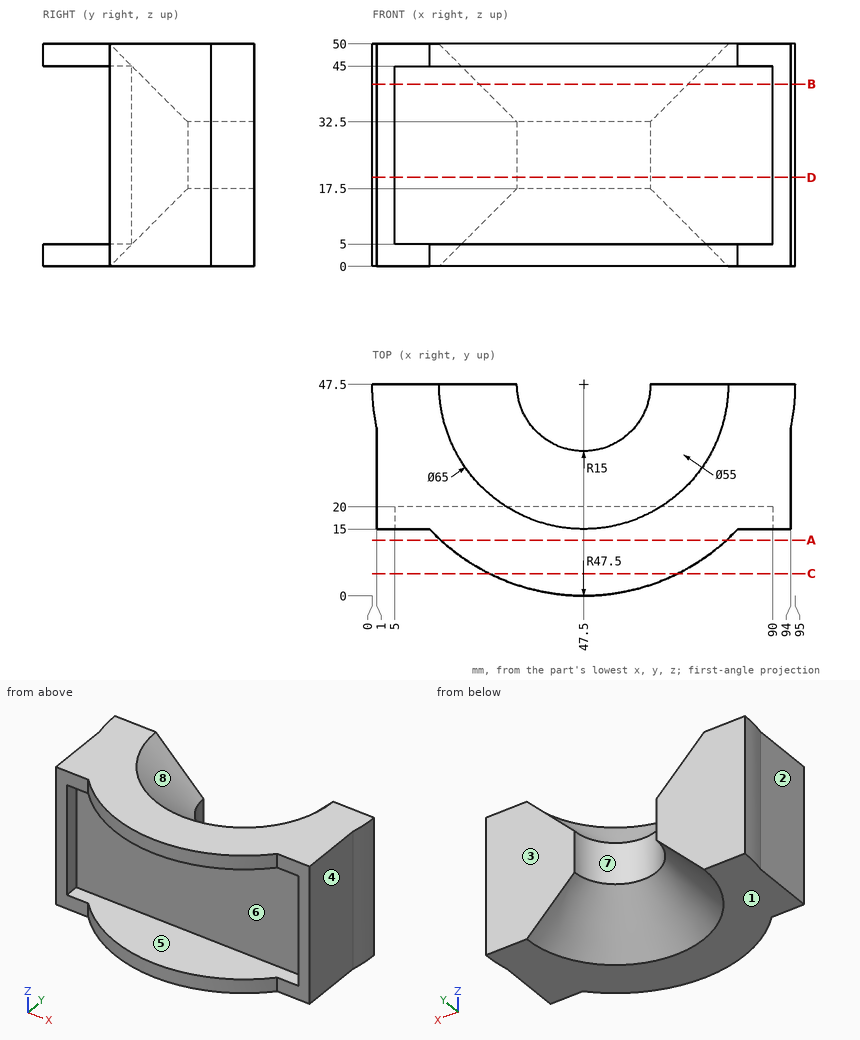
The figure shows three views and two pictorial views of one solid part (mm, origin at its lowest corner). Answer the questions. A direction names the side the tool comes from. Give positions to 0.01 mm unless a question says otherwise; leave off trailing zeros. Loops run counter-clockwise (first coordinate to the right, second up) from the corner with the lowest first, then second, coordinate; pieces in that order, holes last. Notation, with made-up numbers: (40, -14) -> (69, -14) arc R21 cw to (69, -1) -> close; hole circle Ø1 at (-9.5, 60). An arc over 180 degrees is marked (long way). Put each result on its own line as item: value. Start each with the question number.
Item 1: Find the intervals of material crossed by L1, parallel to X at y = 15.5, z = 33; L2, parallel to Z at x = 55, y = 5; L3, parallel to Y at x = 11, z = 40.5, in increasing order. Write a range as [from, to].
Item 2: Each of these flat-tipped pins is pushed along its axis until it touches: P1, Ø25, axis at y = 22.5, z = 37, coming from the -X side; P2, Ø3, axis at x = 12.5, z = 23, coming from the -Y side; P3, Ø6, axis at x = 60.5, y = 35, coming from the +Z side; P4, Ø8, axis at x = 13, y = 6, coming from the -Z side. Where does it stop, or does it pass through?
Item 3: The part is cut by section A-A (y = 12.5). Give the vertices of the cut face in (x, z), then the cut area to 3 significant figures.
Item 4: The part is cut by section D-D (z = 20). Give the vertices of the cut face in (x, y).
Item 5: The part is cut by section C-C (y = 5). Give the vertices of the cut face in (x, z), then the cut area to 3 significant figures.
Item 6: Which of the six approach directions +Z, -Z, +X, -X, +Y, -Y give full straight-line access (tool end or side, diameter ignored) to the marked faces 1, 2, 3, 4 and 5?
Item 7: The part is cut by section B-B (z = 41). Give the vertices of the cut face in (x, y), then the cut area to 3 significant figures.
Item 8: The mould has two halves that part along Z. Classify the marked faces 6, 7 and 8: released by +Z, released by -Z, zero draft, split by the parting line, or undercut.
Answers below:
1. L1: [1, 5], [90, 94]
1. L2: [0, 5], [45, 50]
1. L3: [20, 47.5]
2. P1: x = 1
2. P2: y = 20
2. P3: z = 38.53
2. P4: through
3. outline: (15.39, 0) -> (79.61, 0) -> (79.61, 5) -> (15.39, 5) -> close; (15.39, 45) -> (79.61, 45) -> (79.61, 50) -> (15.39, 50) -> close
3. area: 642 mm2
4. outline: (0, 47.5) arc R47.5 ccw to (1, 37.8) -> (1, 15) -> (5, 15) -> (5, 20) -> (90, 20) -> (90, 15) -> (94, 15) -> (94, 37.8) arc R47.5 ccw to (95, 47.5) -> (62.5, 47.5) arc R15 cw to (32.5, 47.5) -> close
5. outline: (26.29, 0) -> (68.71, 0) -> (68.71, 5) -> (26.29, 5) -> close; (26.29, 45) -> (68.71, 45) -> (68.71, 50) -> (26.29, 50) -> close
5. area: 424 mm2
6. face 1: -Z, +X, -X, +Y, -Y
6. face 2: +Z, -Z, -X, -Y
6. face 3: +Z, -Z, +X, -X, +Y
6. face 4: +Z, -Z, +X, -Y
6. face 5: -Y
7. outline: (0, 47.5) arc R47.5 ccw to (1, 37.8) -> (1, 15) -> (5, 15) -> (5, 20) -> (90, 20) -> (90, 15) -> (94, 15) -> (94, 37.8) arc R47.5 ccw to (95, 47.5) -> (71, 47.5) arc R23.5 cw to (24, 47.5) -> close
7. area: 1,740 mm2
8. face 6: undercut
8. face 7: zero draft
8. face 8: released by +Z
